Check sheet for the modelled part. Datum: model origin and axes. Units: mm. Face numbers are marked on the shaded views. Coordinates: 2 decimals unless noted, no trailing zeros. Loops run counter-clockwise (first coordinate to the right, second up) from the corner with the lowest first, then second, coordinate; pieces in that order, holes last.
```python
from build123d import *

# Parameters (mm, degrees)
BASPROSKE_W         = 6
BASPROSKE_H         = 7.5
TOOTHCUT_DEPTH      = 13.186057607
TEETHCUTS_COUNT     = 10
TEETHCUTS_ANGLE     = 324
BORSKE_R            = 2.5
BORE_DEPTH          = 50.0000508
SKETCH1_R           = 2.6
CUT_EXTRUDE1_DEPTH  = 12.991156361
BOSS_EXTRUDE1_DEPTH = 6


with BuildPart() as part:
    # BasProSke → Base-Revolve (revolve)
    with BuildSketch(Plane(origin=(0, 0, 0), x_dir=(1, 0, 0), z_dir=(0, 1, 0)), mode=Mode.PRIVATE) as base_revolve_sk:
        with Locations((3, 3.75)):
            Rectangle(BASPROSKE_W, BASPROSKE_H)
    revolve(base_revolve_sk.sketch.rotate(Axis((-10, 0, 0), (1, 0, 0)), 180), axis=Axis((-10, 0, 0), (1, 0, 0)))

    # TooCutSke → ToothCut (cut, through all)
    with BuildSketch(Plane(origin=(0, 0, 0), x_dir=(0, 0, -1), z_dir=(1, 0, 0))):
        with BuildLine():
            ThreePointArc((0.737676151, 4.628079099), (0, 4.6865), (-0.737676151, 4.628079099))
            ThreePointArc((-0.737676151, 4.628079099), (-1.051542781, 6.151798382), (-2.205760267, 7.194877817))
            ThreePointArc((-2.205760267, 7.194877817), (0, 7.5254), (2.205760267, 7.194877817))
            ThreePointArc((2.205760267, 7.194877817), (1.051542781, 6.151798382), (0.737676151, 4.628079099))
        make_face()
    toothcut = extrude(amount=TOOTHCUT_DEPTH, mode=Mode.SUBTRACT)

    # TeethCuts: ToothCut ×10 about axis
    teethcuts_axis = Axis((-10, 0, 0), (1, 0, 0))
    for i in range(1, TEETHCUTS_COUNT):
        add(toothcut.rotate(teethcuts_axis, i * TEETHCUTS_ANGLE / (TEETHCUTS_COUNT - 1)), mode=Mode.SUBTRACT)

    # BorSke → Bore (cut, symmetric)
    with BuildSketch(Plane(origin=(0, 0, 0), x_dir=(0, 0, -1), z_dir=(1, 0, 0))):
        with Locations(Location((0, 0, 0), (0, 0, 180))):
            Circle(BORSKE_R)
    extrude(amount=BORE_DEPTH, both=True, mode=Mode.SUBTRACT)

    # Sketch1 → Cut-Extrude1 (cut, through all)
    with BuildSketch(Plane(origin=(6, 0, 0), x_dir=(0, 0, -1), z_dir=(1, 0, 0))):
        Circle(SKETCH1_R)
    extrude(amount=-CUT_EXTRUDE1_DEPTH, mode=Mode.SUBTRACT)

    # Sketch2 → Boss-Extrude1 (add)
    with BuildSketch(Plane(origin=(6, 0, 0), x_dir=(0, 0, -1), z_dir=(1, 0, 0))):
        Polygon((0, 2.6), (2.6, 0), (2.6, 2.6), align=None)
    extrude(amount=-BOSS_EXTRUDE1_DEPTH)


solid = part.part
```
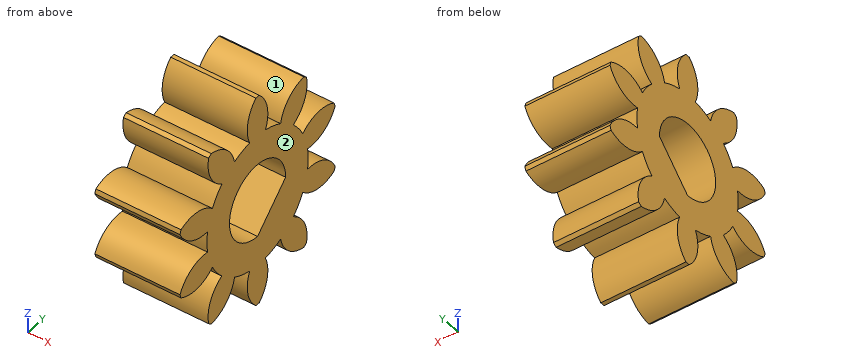
1) Depth check by flat-ended pin: pin 1 (1 mm diameter, centred on x = 5, z = -1, fed in from +Y); pin 2 (2 mm diameter, centred on x = 3, z = -5.5, fed in from -Y). Enter the tip coordinate at first touch or a pass-through.
Answer sheet:
pin 1: stops at y = 6.72
pin 2: stops at y = -4.58
2) Section check A-A on y = 6.75. Enter the section's corners in (x, z), plus the area to 3 significant figures.
Answer sheet:
outline: (0, -2.62) - (6, -2.62) - (6, -1.53) - (0, -1.53) - close; (0, 1.53) - (6, 1.53) - (6, 2.62) - (0, 2.62) - close
area: 13.1 mm2
3) Section check C-C on y = -4. Enter the section's corners in (x, z), plus the area to 3 significant figures.
Answer sheet:
outline: (0, -6.11) - (6, -6.11) - (6, -3.89) - (0, -3.89) - close; (0, -2.44) - (6, -2.44) - (6, 2.44) - (0, 2.44) - close; (0, 3.89) - (6, 3.89) - (6, 6.11) - (0, 6.11) - close
area: 55.9 mm2
4) Mould release check, pull along Y, two halves, no side actions. Record for the marked faces 1 and 2: +Y half, -Y half, draft (parallel to the pull), parting line (faces both ways), or undercut.
Answer sheet:
face 1: undercut
face 2: draft
5) Scan lines: line 1 (Y direction, x = 2.5, z = 5.25); line 2 (Z direction, x = 4.3, y = 4); line 3 (Y direction, x = 1.3, z = 2). Record each from-to range of solid material in increasing order.
Answer sheet:
line 1: y = -4.57 to -2.64, -0.92 to 0.92, 2.64 to 4.57
line 2: z = -6.11 to -3.89, -2.44 to 2.44, 3.89 to 6.11
line 3: y = -7.09 to -1.66, 1.66 to 7.09
6) Section check B-B on z = 5. Enter the section's corners in (x, y).
Answer sheet:
outline: (0, -4.53) - (6, -4.53) - (6, -2.46) - (0, -2.46) - close; (0, -0.86) - (6, -0.86) - (6, 0.86) - (0, 0.86) - close; (0, 2.46) - (6, 2.46) - (6, 4.53) - (0, 4.53) - close
